Source: CAD feature listing. Evaluate the final solid. Frame: model axes, mm. A direction names the side the tool comes from. Give positions to 0.01 mm unless a question says otherwise; leave off trailing zeros. Write each loop counter-clockwise with the first axis right and the second up, starting at its lowest first coordinate (ties: lowest second). Pieces come first, ordered by that corner, then holes. Notation, with made-up numbers: M -23,85 L 13,85 A11 ccw 13,99 Z; hole C 35.5,63 d1. An arc over 180 degrees is marked long. Use CSV: the item, a comma, the result in double quotes. Start each with the question number.
Autodesk Inventor part; units mm, degrees
ref_plane "Start plane" through (0, 0, 20.9785) normal (0, 0, 1) x (1, 0, 0)
ref_plane "End plane" through (0, 0, 265.0285) normal (0, 0, 1) x (1, 0, 0)
ref_plane "Work Plane4" through (9, -130.3465, -77.6904) normal (0, 0.5944, -0.8042) x (1, 0, 0)
ref_plane "Start plane" through (0, 0, 20.9785) normal (0, 0, 1) x (1, 0, 0)
ref_plane "End plane" through (0, 0, 265.0285) normal (0, 0, 1) x (1, 0, 0)
sketch "Sketch" plane through (0, 0, 0) normal (0, 0, 1) x (1, 0, 0)
  line L0 (-15, -9) -> (-15, 9)
  line L1 (-9, 15) -> (9, 15)
  line L2 (15, 9) -> (15, -9)
  line L3 (9, -15) -> (-9, -15)
  arc A0 (-15, -9) -> (-9, -15) centre (-9, -9) ccw
  arc A1 (-9, 15) -> (-15, 9) centre (-9, 9) ccw
  arc A2 (15, 9) -> (9, 15) centre (9, 9) ccw
  arc A3 (9, -15) -> (15, -9) centre (9, -9) ccw
  arc A4 (-9, 12) -> (-12, 9) centre (-9, 9) ccw
  line L4 (-9, 12) -> (9, 12)
  arc A5 (12, 9) -> (9, 12) centre (9, 9) ccw
  line L5 (12, 9) -> (12, -9)
  arc A6 (9, -12) -> (12, -9) centre (9, -9) ccw
  line L6 (9, -12) -> (-9, -12)
  arc A7 (-12, -9) -> (-9, -12) centre (-9, -9) ccw
  line L7 (-12, -9) -> (-12, 9)
  line L8 (0, 22.7397) -> (0, -22.7397) construction
  line L9 (-22.7397, 0) -> (22.7397, 0) construction
  dimension "d7" = 6
  dimension "d10" = 30
  dimension "d11" = 30
  dimension "d12" = 3
  dimension "d15" = 15
  dimension "d16" = 15
extrude "Body" add sketch "Sketch" along normal up to surface (244.05 mm away) from surface at 20.9785
sketch "Sketch3" plane through (0, 0, 0) normal (0, 0, 1) x (1, 0, 0)
  line L0 (0, 0) -> (10, 0)
ref_plane "Work Plane3" through (0, 0, 0) normal (0, -1, 0) x (1, 0, 0)
ref_plane "Work Plane4" through (9, -130.3465, -77.6904) normal (0, 0.5944, -0.8042) x (1, 0, 0)
split "Split1" plane through (9, -130.3465, -77.6904) removes the side toward (0, 0.5944, -0.8042)
ref_plane "Work Plane5" through (9, -433.7307, 612.048) normal (0, -0.8042, -0.5944) x (1, 0, 0)
split "Split2" plane through (9, -433.7307, 612.048) removes the side toward (0, -0.8042, -0.5944)
ref_plane "Work Plane6" through (-9, -321.146, 695.2627) normal (0, 0.8042, 0.5944) x (1, 0, 0)
split "Split3" plane through (-9, -321.146, 695.2627) removes the side toward (0, 0.8042, 0.5944)
ref_plane "Work Plane7" through (9, 8.9159, 273.9444) normal (0, -0.5944, 0.8042) x (1, 0, 0)
split "Split4" plane through (9, 8.9159, 273.9444) removes the side toward (0, -0.5944, 0.8042)
sketch "Sketch4" plane through (0, 0, 0) normal (0, -1, 0) x (1, 0, 0)
  line L0 (-2, 20.9785) -> (12, 20.9785)
  line L1 (-2, 265.0285) -> (12, 265.0285)
  dimension "d18" = 244.05
equation "\"d7\" = G_IR"
equation "\"d10\" = G_H"
equation "\"d11\" = G_W"
equation "\"d12\" = G_T"
equation "\"d15\" = 0.5 * d10"
equation "\"d16\" = 0.5 * d11"
equation "\"d3\" = G_L"
equation "\"G_W\" = 30"
equation "\"G_H\" = 30"
equation "\"G_T\" = 3"
equation "\"G_IR\" = 6"
equation "\"G_L\" = d18"
equation "\"G_OFFSET_START\" = -20.97851"
equation "\"G_OFFSET_END\" = -20.97851"
equation "\"d13\" = -G_OFFSET_START"
equation "\"d14\" = G_OFFSET_END + B_L"
equation "\"B_L\" = 286.00699"
properties part number "DIN EN 10219-2 - 30 x 30 x 3  - 244.05" material "Steel, Mild"
1. Section C-C on z = 148.5. Return loops of the section in (x, y), then the cut area to 3 significant figures.
2. Line query: probe 1 along Y at (x, z) = (3.5, 51); probe 2 along Y at (x, z) = (-11, 103). Output: solid intervals per line, ascending.
3. Section B-B on x = 6.75. Return loops of the section in (y, z), then the cut area to 3 significant figures.
4. First-contact query: pin 1 (2 mm diameter, centred on x = -11, z = 51.5, fed in from +Y). Flat tip, straight axial feed; report the tip coordinate or a pass-through.
5. Section A-A on y = -1. Return loops of the section in (x, z), then the cut area to 3 significant figures.
6. Access query for faces 4 (the flat face through (0, -12, 148)), 5 (the flat face through (1.041, -12.606, 42.283)). Directions: +Z, -Z, +X, -X, +Y, -Y. A direction counts if a zero-diameter tool reaches every point of the face in a straight line with its end or side. Return the directions, or none.
7. Pull-direction query (X, two-part tool) for faces 1 (the flat face through (0, 12, 135)), 2 (the cylindrical face through (-13.289, 13.196, 135.383)), 3 (the cylindrical face through (13.289, -13.196, 147.49)); classes: released by +X, released by -X, zero draft, split by the parting line, or undercut.
Resolved:
1,outline,"M -15,-9 A6 ccw -9,-15 L 9,-15 A6 ccw 15,-9 L 15,9 A6 ccw 9,15 L -9,15 A6 ccw -15,9 Z; hole M -12,-9 A3 ccw -9,-12 L 9,-12 A3 ccw 12,-9 L 12,9 A3 ccw 9,12 L -9,12 A3 ccw -12,9 Z"
1,area,"301 mm2"
2,probe 1,"y = -15 to -12, 12 to 15"
2,probe 2,"y = -14.66 to -11.24, 11.24 to 14.66"
3,outline,"M -15,45.52 L -12,41.46 L -12,258.49 L -15,256.27 Z; M 12,27.52 L 15,29.74 L 15,240.47 L 12,244.53 Z"
3,area,"1,280 mm2"
4,pin 1,"stops at y = 14.92"
5,outline,"M -15,26.58 L -12,26.58 L -12,262.12 L -15,262.12 Z; M 12,26.58 L 15,26.58 L 15,262.12 L 12,262.12 Z"
5,area,"1,410 mm2"
6,face 4,"+Z, -Z"
6,face 5,"-Z, +X, -X, -Y"
7,face 1,"undercut"
7,face 2,"released by -X"
7,face 3,"released by +X"
